The model under review builds one solid part; all positions refer to its coordinate system, in mm. Face numbers are marked on the shaded views. A direction names the side the tool comes from. Give positions to 0.01 mm unless a question says otherwise; leave off trailing zeros. Loops run counter-clockwise (first coordinate to the right, second up) from the corner with the lowest first, then second, coordinate; pieces in that order, holes last. Notation, with made-up numbers: M -1,32 L 23,32 A18 cw 23,57 Z; hole C 28.5,6.5 d2. An arc over 180 degrees is marked long. One line per item, written item: value. Start each with the question number.
Q1. For the marked faces 5 and 6, list the 3-axis set-ups (+Z, -Z, +X, -X, +Y, -Y) from which the entire face can be reached by the end or side of a thin tool; tool diameter is ignored.
Q2. To check wall thickness, follow line 1 along Y through (x, z) = (-9, 15) (3 decimals); line 2 along X through (y, z) = (-6.5, 30) (3 decimals); line 3 along Z through (x, y) = (1.5, -60) (3 decimals). State the ranges of each line that lie inside material, in increasing order. Write a range as from..to.
Q3. We need section B-B on z = 51.5. Write out the cut boundary in (x, y) (3 decimals).
Q4. We need section C-C on x = 8.5. Write out the cut boundary in (y, z) (3 decimals), plus the area to 3 significant figures.
Q5. We need section A-A on y = -15. Write out the cut boundary in (x, z) (3 decimals).
Q6. Mouldability with a two-part tool opening along X and no side actions: class the marked faces 1, 2, 3 and 4 as released by +X, released by -X, zero draft, split by the parting line, or undercut.
```python
from build123d import *

# Parameters (mm, degrees)
F0_W     = 57.15
F0_H     = 57.15
F1_DEPTH = 3.175
F2_DEPTH = 63.5
F0_W_2   = 3.175
F0_H_2   = 3.175
F3_DEPTH = 63.5
F4_DEPTH = 63.5
F5_DEPTH = 63.5


with BuildPart() as f1:
    # F0 (on Top) → F1 (new body)
    with BuildSketch(Plane.XY):
        with Locations((0, -31.75)):
            Rectangle(F0_W, F0_H)
    extrude(amount=F1_DEPTH)

    # F0 (on Top) → F2 (join)
    with BuildSketch(Plane.XY):
        Polygon((31.75, 0), (-31.75, 0), (-31.75, -3.175), (-28.575, -3.175), (28.575, -3.175), (31.75, -3.175), align=None)
    extrude(amount=F2_DEPTH)

    # F0 (on Top) → F3 (join)
    with BuildSketch(Plane.XY):
        with Locations((-30.1625, -31.75)):
            Rectangle(F0_W_2, F0_H)
        with Locations((-30.1625, -61.9125)):
            Rectangle(F0_W_2, F0_H_2)
    extrude(amount=F3_DEPTH)

    # F0 (on Top) → F4 (join)
    with BuildSketch(Plane.XY):
        Polygon((31.75, -63.5), (31.75, -60.325), (28.575, -60.325), (-28.575, -60.325), (-28.575, -63.5), align=None)
    extrude(amount=F4_DEPTH)

    # F0 (on Top) → F5 (join)
    with BuildSketch(Plane.XY):
        with Locations((30.1625, -31.75)):
            Rectangle(F0_W_2, F0_H)
    extrude(amount=F5_DEPTH)


solid = f1.part
```
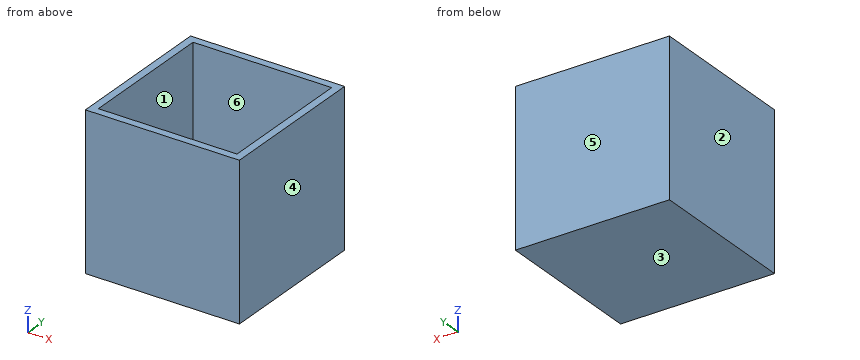
Solved:
1. face 5: +Z, -Z, +X, -X, +Y
1. face 6: +Z
2. line 1: -63.5..-60.325, -3.175..0
2. line 2: -31.75..-28.575, 28.575..31.75
2. line 3: 0..3.175
3. outline: M -31.75,-63.5 L 31.75,-63.5 L 31.75,0 L -31.75,0 Z; hole M -28.575,-60.325 L 28.575,-60.325 L 28.575,-3.175 L -28.575,-3.175 Z
4. outline: M -63.5,0 L 0,0 L 0,63.5 L -3.175,63.5 L -3.175,3.175 L -60.325,3.175 L -60.325,63.5 L -63.5,63.5 Z
4. area: 585 mm2
5. outline: M -31.75,0 L 31.75,0 L 31.75,63.5 L 28.575,63.5 L 28.575,3.175 L -28.575,3.175 L -28.575,63.5 L -31.75,63.5 Z
6. face 1: undercut
6. face 2: released by -X
6. face 3: zero draft
6. face 4: released by +X
